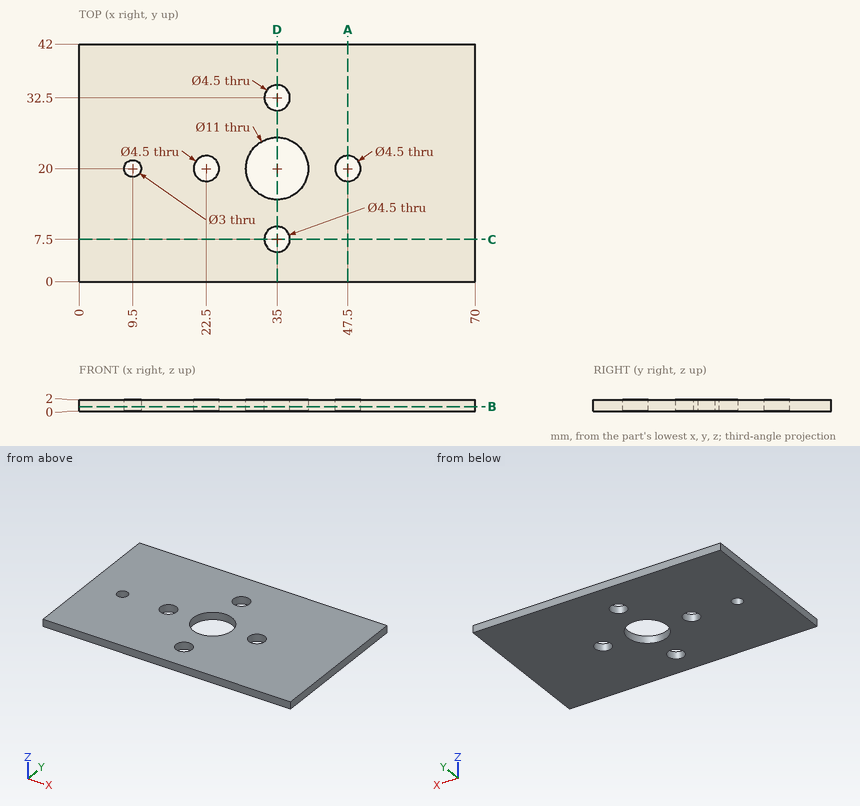
Study the drawing (mm; zero at the part's minimum x, y, z) and answer. Coordinates: 2 decimals unless noted, no trailing zeros. Write each loop counter-clockwise with the first axis right and the second up, starting at its lowest first coordinate (ties: lowest second). Pieces come first, ordered by that corner, then holes. Notation, with made-up numbers: (-37.5, 76.25) - (-13.5, 76.25) arc R21 ccw to (-13.5, 96.25) - close; hole circle Ø10 at (37.25, -26.75). An arc over 180 degrees is marked (long way). Put each result on its own line as item: value.
1. Find the intervals of material crossed by line 1 along Y through (x, z) = (35, 1.1); line 2 along Y through (x, z) = (22.5, 1.5); line 3 along Y through (x, z) = (33, 1.85), in increasing order. Write a range as from..to.
Answer sheet:
line 1: y = 0..5.25, 9.75..14.5, 25.5..30.25, 34.75..42
line 2: y = 0..17.75, 22.25..42
line 3: y = 0..6.47, 8.53..14.88, 25.12..31.47, 33.53..42
2. The part is cut by section D-D on x = 35. Give the vertices of the cut face in (y, z), plus the area to 3 significant figures.
Answer sheet:
outline: (0, 0) - (5.25, 0) - (5.25, 2) - (0, 2) - close; (9.75, 0) - (14.5, 0) - (14.5, 2) - (9.75, 2) - close; (25.5, 0) - (30.25, 0) - (30.25, 2) - (25.5, 2) - close; (34.75, 0) - (42, 0) - (42, 2) - (34.75, 2) - close
area: 44.0 mm^2
3. The part is cut by section C-C on y = 7.5. Give the vertices of the cut face in (x, z).
Answer sheet:
outline: (0, 0) - (32.75, 0) - (32.75, 2) - (0, 2) - close; (37.25, 0) - (70, 0) - (70, 2) - (37.25, 2) - close
4. The part is cut by section A-A on x = 47.5. Give the vertices of the cut face in (y, z).
Answer sheet:
outline: (0, 0) - (17.75, 0) - (17.75, 2) - (0, 2) - close; (22.25, 0) - (42, 0) - (42, 2) - (22.25, 2) - close
5. The part is cut by section B-B on z = 0.8. Give the vertices of the cut face in (x, y), plus the area to 3 significant figures.
Answer sheet:
outline: (0, 0) - (70, 0) - (70, 42) - (0, 42) - close; hole circle Ø3 at (9.5, 20); hole circle Ø4.5 at (22.5, 20); hole circle Ø11 at (35, 20); hole circle Ø4.5 at (35, 7.5); hole circle Ø4.5 at (35, 32.5); hole circle Ø4.5 at (47.5, 20)
area: 2,770 mm^2
6. Flat-ended cylindrical pins translate along their axes: pin 1 Ø2.5 at (x, y) = (35, 32.5) entering from +Z; pin 2 Ø17.5 at (x, y) = (35, 20) entering from -Z. Find the tip coordinate at first contact, or state that the pin passes through.
Answer sheet:
pin 1: passes through
pin 2: stops at z = 0
